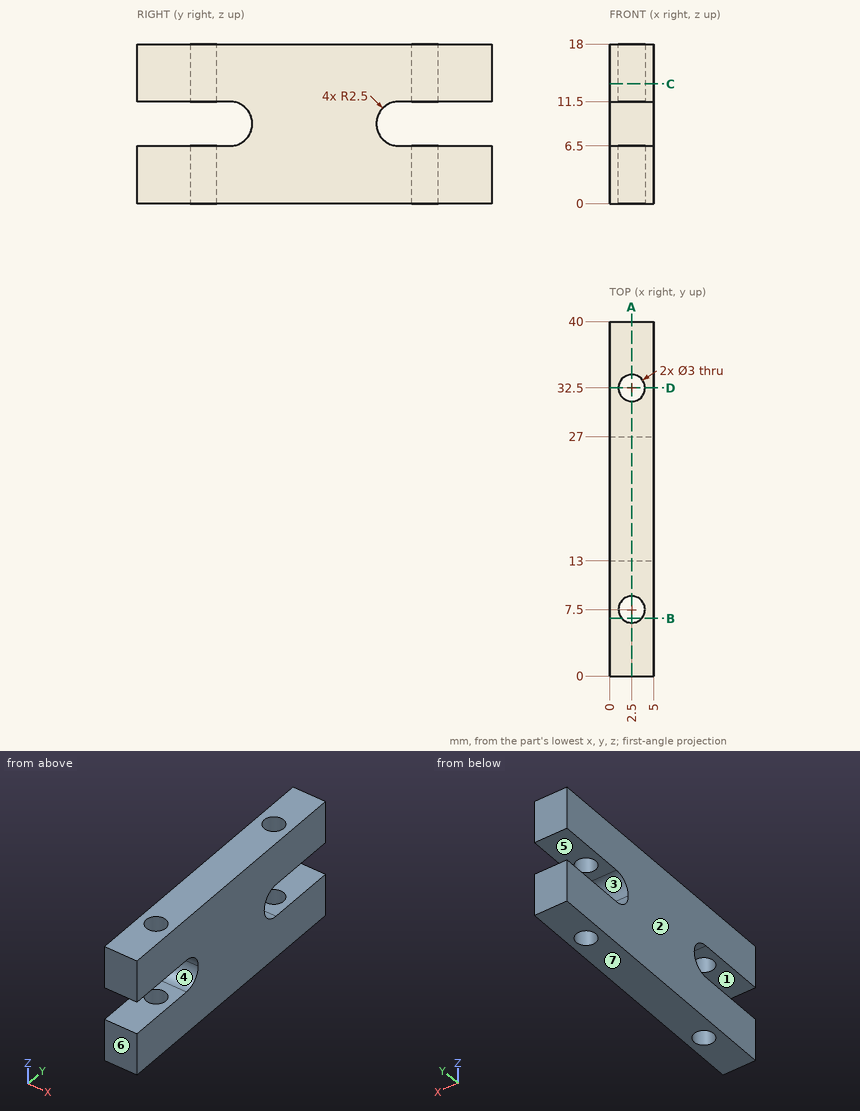
Study the drawing (mm; zero at the part's minimum x, y, z) and answer. A direction names the side the tool comes from. Round coordinates to 2 decimals unless told otherwise and drop trailing zeros. Write each loop counter-clockwise with the first axis right and the second up, starting at its lowest first coordinate (ties: lowest second). Pieces come first, ordered by that corner, then holes. Notation, with made-up numbers: (-12.5, 4.25) -> (30.5, 4.25) arc R33 ccw to (30.5, 33.25) -> close; hole circle Ø3 at (76.5, 3). An arc over 180 degrees is marked (long way). Write each question's results on one line, items separated by ' | '.
Item 1: A cutting plane is placed at A-A, the plane x = 2.5. Count the separate pieces of the cut face and the enclosed holes in it, plus the area to 3 significant figures.
Result set:
separate pieces: 5 | enclosed holes: 0 | area: 517 mm^2
Item 2: Find the intervals of material crossed by line 1 along Z through (x, y) = (1.1, 35.5); line 2 along X through (y, z) = (7.5, 15.5); line 3 along Y through (x, z) = (1.2, 12.25), in increasing order. Write a range as [from, to].
Result set:
line 1: [0, 6.5], [11.5, 18] | line 2: [0, 1], [4, 5] | line 3: [0, 6.75], [8.25, 31.75], [33.25, 40]
Item 3: A cutting plane is placed at D-D, the plane y = 32.5. Determine the outline of the cut face in (x, z), plus the area to 3 significant figures.
Result set:
outline: (0, 0) -> (1, 0) -> (1, 6.5) -> (0, 6.5) -> close; (0, 11.5) -> (1, 11.5) -> (1, 18) -> (0, 18) -> close; (4, 0) -> (5, 0) -> (5, 6.5) -> (4, 6.5) -> close; (4, 11.5) -> (5, 11.5) -> (5, 18) -> (4, 18) -> close | area: 26.0 mm^2
Item 4: A cutting plane is placed at C-C, the plane z = 13.5. Determine the outline of the cut face in (x, y), plus the area to 3 significant figures.
Result set:
outline: (0, 0) -> (5, 0) -> (5, 40) -> (0, 40) -> close; hole circle Ø3 at (2.5, 7.5); hole circle Ø3 at (2.5, 32.5) | area: 186 mm^2
Item 5: Which of the six approach directions +Z, -Z, +X, -X, +Y, -Y give full straight-line access (tool end or side, diameter ignored) to the marked faces 1, 2 and 3?
Result set:
face 1: +X, -X, -Y | face 2: +Z, -Z, -X, +Y, -Y | face 3: +X, -X, +Y
Item 6: The mould has two halves that part along Z. Classify the marked faces 4, 5, 6 and 7: +Z half, -Z half, draft (parallel to the pull), parting line (faces both ways), or undercut.
Result set:
face 4: undercut | face 5: undercut | face 6: draft | face 7: -Z half
Item 7: Flat-ended cylindrical pins translate along their axes: P1, Ø2.5, axis at x = 2.5, y = 32.5, coming from the -Z side; P2, Ø2.5, axis at x = 3.5, y = 4.5, coming from the -Z side. Find the tip coordinate at first contact, or state that the pin passes through.
Result set:
P1: through | P2: z = 0
Item 8: A cutting plane is placed at B-B, the plane y = 6.5. Determine the outline of the cut face in (x, z), plus the area to 3 significant figures.
Result set:
outline: (0, 0) -> (1.38, 0) -> (1.38, 6.5) -> (0, 6.5) -> close; (0, 11.5) -> (1.38, 11.5) -> (1.38, 18) -> (0, 18) -> close; (3.62, 0) -> (5, 0) -> (5, 6.5) -> (3.62, 6.5) -> close; (3.62, 11.5) -> (5, 11.5) -> (5, 18) -> (3.62, 18) -> close | area: 35.9 mm^2
